from build123d import *

# Parameters (mm, degrees)
SKETCH1_R           = 100
BOSS_EXTRUDE1_DEPTH = 9
SKETCH2_R           = 7
BOSS_EXTRUDE2_DEPTH = 13
FILLET1_R           = 2


with BuildPart() as part:
    # Sketch1 → Boss-Extrude1 (new body)
    with BuildSketch(Plane(origin=(0, 0, 0), x_dir=(1, 0, 0), z_dir=(0, 1, 0))):
        Circle(SKETCH1_R)
    extrude(amount=BOSS_EXTRUDE1_DEPTH)

    # Sketch2 → Boss-Extrude2 (add)
    with BuildSketch(Plane(origin=(0, 9, 0), x_dir=(1, 0, 0), z_dir=(0, 1, 0))):
        Circle(SKETCH2_R)
    extrude(amount=BOSS_EXTRUDE2_DEPTH)

    # Fillet1
    fillet1_edges = [part.edges().sort_by_distance(p)[0] for p in [
        (-100, 9, 0),
        (-7, 22, 0),
    ]]
    fillet(fillet1_edges, radius=FILLET1_R)


solid = part.part
Here's how the part is built. I have some questions about the finished solid (model axes, mm). A direction names the side the tool comes from. Round coordinates to 2 decimals unless told otherwise and drop trailing zeros. Loops run counter-clockwise (first coordinate to the right, second up) from the corner with the lowest first, then second, coordinate; pieces in that order, holes last. Notation, with made-up numbers: (40.25, 24.5) - (75.25, 24.5) arc R23 ccw to (75.25, 52.5) - close; hole circle Ø2 at (19.5, 4.25). An arc over 180 degrees is marked (long way). One line per question, with ' | ' between items. Start each with the question number.
Q1. I want a section at C-C (y = 16.5). Write out the boundary of the cut face in (x, z).
Q2. Will these pins go through, and if not, where does the flat tip stop? pin 1 (8 mm diameter, centred on x = 16.5, y = 2, fed in from +Z); pin 2 (1 mm diameter, centred on x = 54.5, z = 15, fed in from +Y); pin 3 (12 mm diameter, centred on x = -37.5, z = 0.5, fed in from -Y); pin 4 (12 mm diameter, centred on x = 79, y = 3.5, fed in from +Z).
Q3. Please list where these lines run through material, in increasing order: line 1 (Y direction, x = -37.5, z = -67); line 2 (X direction, y = 2, z = 2); line 3 (X direction, y = 6, z = 35). Write a range as [from, to].
Q4. For faces 1 (the cylindrical face through (6.466, 14.423, 2.681)), 2 (the flat face through (-1, 0, -1)), which set-ups out of +Z, -Z, +X, -X, +Y, -Y let a thin tool reach every point of the face, with its end or its side?
Q5. I want a section at B-B (x = 0). Write out the boundary of the cut face in (y, z), then the cut area to 3 significant figures.
Q6. I want a section at A-A (z = 0). Write out the boundary of the cut face in (x, y).
Response values:
1) outline: circle Ø14 at (0, 0)
2) pin 1: stops at z = 99.22 | pin 2: stops at y = 9 | pin 3: stops at y = 0 | pin 4: stops at z = 68.34
3) line 1: y = [0, 9] | line 2: x = [-99.98, 99.98] | line 3: x = [-93.67, 93.67]
4) face 1: +Y | face 2: +Z, -Z, +X, -X, -Y
5) outline: (0, -100) - (7, -100) arc R2 ccw to (9, -98) - (9, -7) - (20, -7) arc R2 ccw to (22, -5) - (22, 5) arc R2 ccw to (20, 7) - (9, 7) - (9, 98) arc R2 ccw to (7, 100) - (0, 100) - close | area: 1,980 mm²
6) outline: (-100, 0) - (100, 0) - (100, 7) arc R2 ccw to (98, 9) - (7, 9) - (7, 20) arc R2 ccw to (5, 22) - (-5, 22) arc R2 ccw to (-7, 20) - (-7, 9) - (-98, 9) arc R2 ccw to (-100, 7) - close
